Part print with two shaded views. Sizes in mm from the minimum x, y, z corner. Coordinates: 2 decimals unless noted, no trailing zeros. Write each loop counter-clockwise with the first axis right and the second up, starting at its lowest first coordinate (ties: lowest second). Pieces come first, ordered by that corner, then holes. Notation, with made-up numbers: (54, 58.5) - (66, 58.5) arc R16 cw to (66, 72.5) - close; hole circle Ø7 at (23, -26.75). An arc over 180 degrees is marked (long way). One line per question, with ' | ' between items. Start each with the question number.
1. Band-saw the part on D-D, the plane x = 25. Write the cut outline in (y, z) (3 decimals), then the cut area to 3 significant figures.
2. Probe line 1 (Y direction, x = 68.5, z = 0.25); line 2 (X direction, y = 19, z = 0.65); line 3 (X direction, y = 99, z = 1.9). List the from-to ranges inside material, lowest first.
3. Flat gauge pins, fed straight in: P1, Ø1.5, axis at x = 17.5, z = 2, coming from the -Y side; P2, Ø1.5, axis at x = 53.5, z = 0.5, coming from the -Y side; P3, Ø1.6, axis at x = 55.5, z = 2.5, coming from the -Y side. Where does each tip first touch, or does it go through?
4. Band-saw the part on A-A, the plane x = 41. Write the cut outline in (y, z) (1 decimal), then the cut area to 3 significant figures.
5. Band-saw the part on B-B, the plane y = 118.5. Write the cut outline in (x, z) (3 decimals).
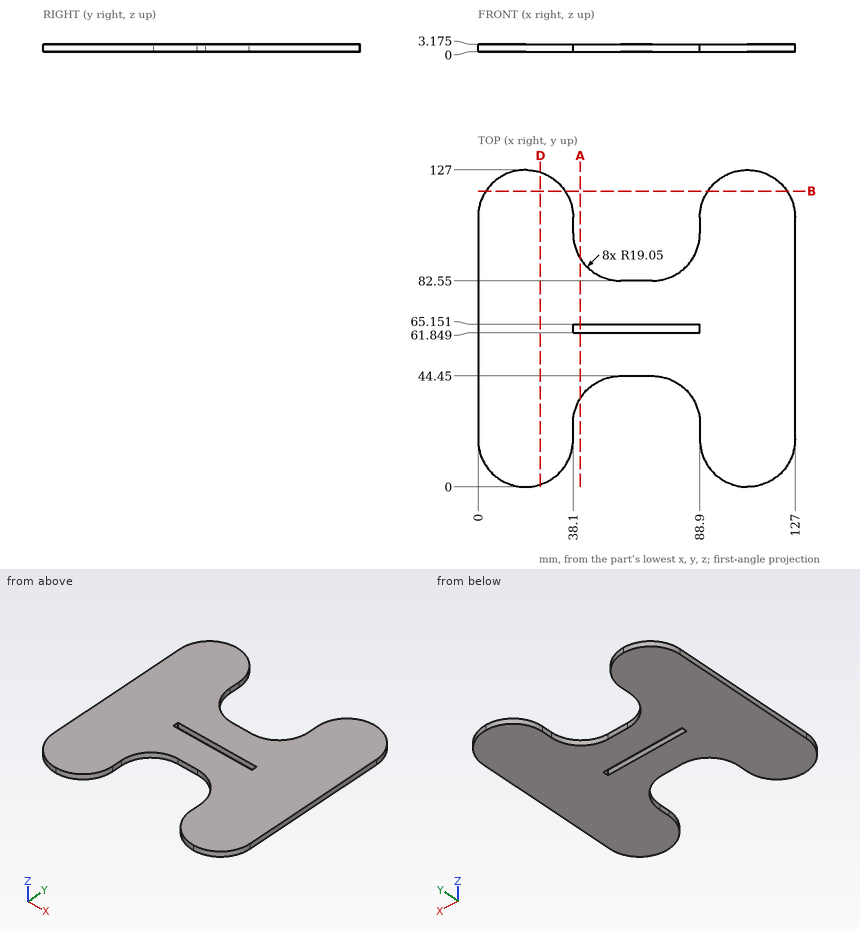
Filled in:
1) outline: (0.953, 0) - (126.047, 0) - (126.047, 3.175) - (0.953, 3.175) - close | area: 397 mm²
2) line 1: y = 44.45 to 61.85, 65.15 to 82.55 | line 2: x = 0 to 38.1, 88.9 to 127 | line 3: x = 0 to 38.28, 88.72 to 127
3) P1: stops at y = 0.02 | P2: stops at y = 43.93 | P3: stops at y = 44.29
4) outline: (35.5, 0) - (61.8, 0) - (61.8, 3.2) - (35.5, 3.2) - close; (65.2, 0) - (91.5, 0) - (91.5, 3.2) - (65.2, 3.2) - close | area: 167 mm²
5) outline: (3.188, 0) - (34.912, 0) - (34.912, 3.175) - (3.188, 3.175) - close; (92.088, 0) - (123.812, 0) - (123.812, 3.175) - (92.088, 3.175) - close
